```python
from build123d import *

# Parameters (mm, degrees)
F2_DEPTH      = 55
F2_DEPTH_BACK = 55


with BuildPart() as f2:
    # F1 (on Right) → F2 (new body, two sides)
    with BuildSketch(Plane.YZ) as f2_sk:
        Polygon((-9.27, -2.5), (-2.5, -2.5), (-3.3021166542, -0.2962026049), align=None)
        Polygon((3.3021166542, -0.2962026049), (2.5, 0), (2.5, -2.5), align=None)
        Polygon((-2.5, 0), (-2.5, 2.5), (-4.3198511713, 2.5), (-3.3021166542, -0.2962026049), align=None)
        Polygon((2.5, -2.5), (-2.5, -2.5), (-9.27, -2.5), (-9.27, -4.5), (9.27, -4.5), (9.27, -2.5), align=None)
        Polygon((2.5, 2.5), (-2.5, 2.5), (-2.5, 0), (-2.5, -2.5), (2.5, -2.5), (2.5, 0), align=None)
        Polygon((4.3198511713, 2.5), (2.5, 2.5), (2.5, 0), (3.3021166542, -0.2962026049), align=None)
        Polygon((-2.5, -2.5), (-2.5, 0), (-3.3021166542, -0.2962026049), align=None)
        Polygon((3.3021166542, -0.2962026049), (2.5, -2.5), (9.27, -2.5), align=None)
    extrude(amount=F2_DEPTH)
    extrude(f2_sk.sketch, amount=-F2_DEPTH_BACK)


solid = f2.part
```
CAD build for the part. Positions are in the model's coordinates, mm. A direction names the side the tool comes from. Round coordinates to 2 decimals unless told otherwise and drop trailing zeros. Order: outer loops, then holes, each group sorted by start corner. A loop starts at its lowest first (then second) coordinate and runs counter-clockwise, first axis right, second up.
Item 1: Mould opens along Z. For faces 3 (the face through (1, 0, -4.5)), 4 (the face through (55, 0, -2)), 5 (the face through (0.77, 3.804, 1.082)) say: pulls with the +Z half, pulls with the -Z half, needs draft (parallel to the pull), parting line crosses it, or undercut.
Item 2: Saw through at A-A on x = -17.5. Write the cut outline in (y, z).
Item 3: Saw through at B-B on y = -7. Write the cut outline in (x, z).
Item 4: Saw through at C-C on z = -1.5. Write the cut outline in (x, y), then the cut area to 3 significant figures.
Item 5: Probe line 1 along Y through (x, z) = (-9, -0.25); line 2 along Y through (x, z) = (48, 0.5); line 3 along Z through (x, y) = (44.5, -8.5). List the from-to ranges inside material, lowest first.
Item 6: Tool access for faces 1 (the face through (1, 0, 2.5)), 2 (the face through (0.77, -3.818, 1.121)): list every direction of +Z, -Z, +X, -X, +Y, -Y with a clear straight run to the whole face (end or side of a thin tool).
Reported:
1. face 3: pulls with the -Z half
1. face 4: needs draft
1. face 5: undercut
2. outline: (-9.27, -4.5) - (9.27, -4.5) - (9.27, -2.5) - (3.3, -0.3) - (4.32, 2.5) - (-4.32, 2.5) - (-3.3, -0.3) - (-9.27, -2.5) - close
3. outline: (-55, -4.5) - (55, -4.5) - (55, -1.66) - (-55, -1.66) - close
4. outline: (-55, -6.56) - (55, -6.56) - (55, 6.56) - (-55, 6.56) - close
4. area: 1,440 mm2
5. line 1: y = -3.32 to 3.32
5. line 2: y = -3.59 to 3.59
5. line 3: z = -4.5 to -2.22
6. face 1: +Z, +X, -X, +Y, -Y
6. face 2: +X, -X, -Y
